Here's the drawing with two shaded views (mm, measured from the low corner). I have some questions. Coordinates: 2 decimals unless noted, no trailing zeros. Loops run counter-clockwise (first coordinate to the right, second up) from the corner with the lowest first, then second, coordinate; pieces in that order, holes last.
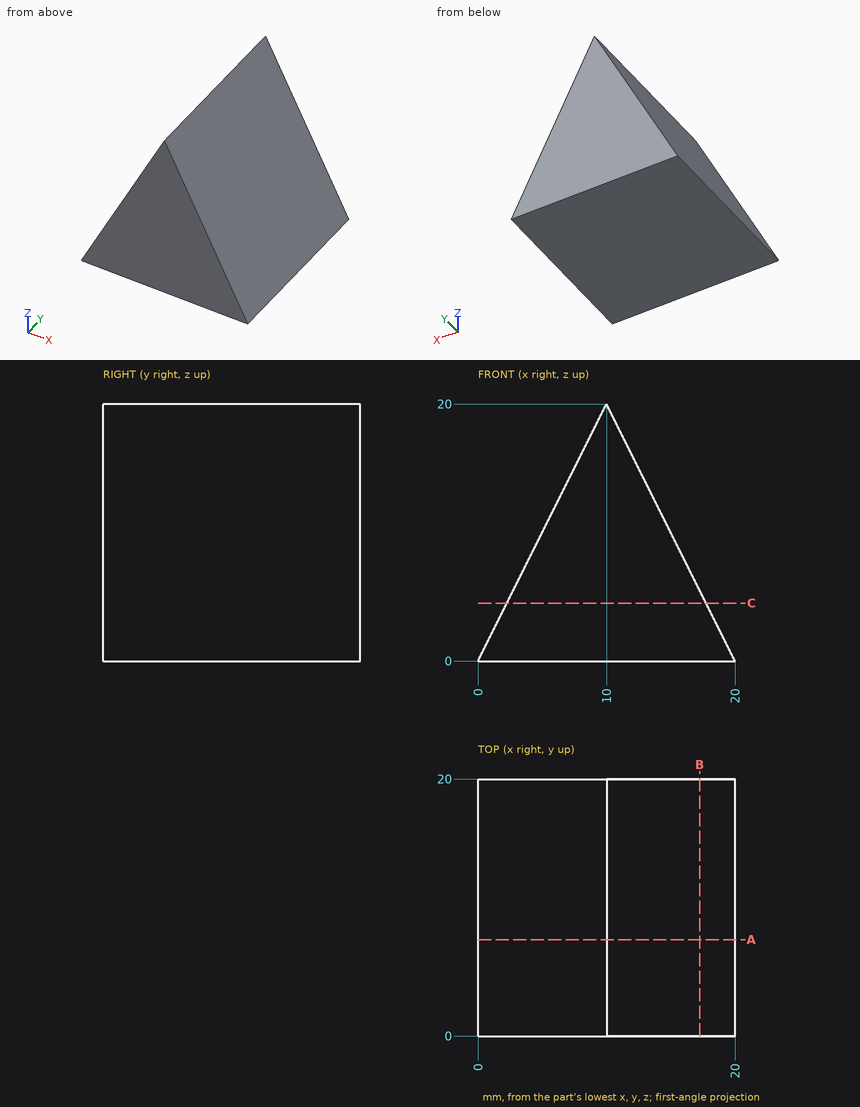
(1) I want a section at B-B on x = 17.25. Write out the boundary of the cut face in (y, z), then the cut area to 3 significant figures.
Check values:
outline: (0, 0) - (20, 0) - (20, 5.5) - (0, 5.5) - close
area: 110 mm2
(2) I want a section at A-A on y = 7.5. Write out the boundary of the cut face in (x, z), then the cut area to 3 significant figures.
Check values:
outline: (0, 0) - (20, 0) - (10, 20) - close
area: 200 mm2
(3) If I drill on probe 1 along X at (y, z) = (2.5, 19); probe 2 along X at (y, z) = (9.5, 18); probe 3 along Z at (x, y) = (19.25, 16.25), over which ranges is the centre line in solid material (lowest first)?
Check values:
probe 1: x = 9.5 to 10.5
probe 2: x = 9 to 11
probe 3: z = 0 to 1.5
(4) I'm going to push flat-ended pins straight in: pin 1 (2 mm diameter, centred on x = 5, y = 16, fed in from +Z); pin 2 (1 mm diameter, centred on y = 16, z = 10, fed in from +X); pin 3 (1.5 mm diameter, centred on y = 5, z = 13.5, fed in from -X) (3 decimals). Where does each tip first touch, or does it pass through?
Check values:
pin 1: stops at z = 12
pin 2: stops at x = 15.25
pin 3: stops at x = 6.375
(5) I want a section at C-C on z = 4.5. Write out the boundary of the cut face in (x, y).
Check values:
outline: (2.25, 0) - (17.75, 0) - (17.75, 20) - (2.25, 20) - close
